Job drawing, mm, ordinate dimensions from the low corner. One solid piece. A direction names the side the tool comes from. Coordinates: 2 decimals unless noted, no trailing zeros. Loops run counter-clockwise (first coordinate to the right, second up) from the corner with the lowest first, then second, coordinate; pieces in that order, holes last. Notation, with made-up numbers: (-39.75, 4) -> (-19.75, 4) arc R12 cw to (-19.75, 24) -> close; hole circle Ø4 at (-22.5, -15). An arc over 180 degrees is marked (long way). Use one line per item in the form item = value. Start each with the question number.
(1) Band-saw the part on D-D on x = 99. Give the cut face in (y, z).
(2) Band-saw the part on C-C on y = 3.25. Give the cut face in (x, z).
(3) Pin check, flat tips, straight feed: P1, Ø6.5, axis at x = 32.5, y = 12.5, coming from the -Z side; P2, Ø5, axis at y = 7, z = 6, coming from the -X side; P3, Ø5, axis at y = 8, z = 2.5, coming from the +X side. Stop position of each tip, or through.
(4) Band-saw the part on B-B on x = 14. Give the cut face in (y, z).
(5) 3-axis set-ups, long thin cutter, end or side, ignore diameter. For the marked faces 1, 2 and 3: which of +Z, -Z, +X, -X, +Y, -Y reach the whole face in a straight line?
(6) Mould opens along X. For the marked faces 4, 5 and 6 say: +X half, -X half, draft (parallel to the pull), parting line (faces both ways), or undercut.
(7) Drill centre lines: L1, parallel to Z at x = 85.5, y = 18.5; L2, parallel to X at y = 15.5, z = 12.75; L3, parallel to Z at x = 104.5, y = 5.25. Where is each one in solid material? Low to high. Write a range as [from, to].
(8) Band-saw the part on A-A on z = 3.75. Give the cut face in (x, y).
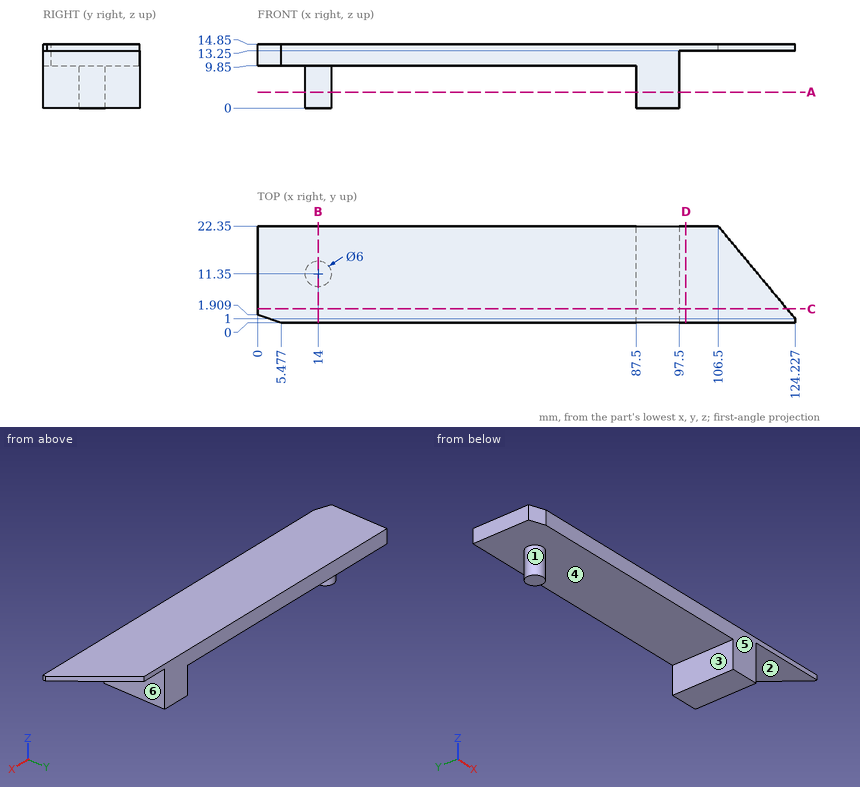
A:
q1.outline = (0, 13.25) -> (22.35, 13.25) -> (22.35, 14.85) -> (0, 14.85) -> close
q2.outline = (0, 9.85) -> (87.5, 9.85) -> (87.5, 0) -> (97.5, 0) -> (97.5, 13.25) -> (122.36, 13.25) -> (122.36, 14.85) -> (0, 14.85) -> close
q3.P1 = 9.85
q3.P2 = 11.64
q3.P3 = 97.5
q4.outline = (0, 9.85) -> (8.35, 9.85) -> (8.35, 0) -> (14.35, 0) -> (14.35, 9.85) -> (22.35, 9.85) -> (22.35, 14.85) -> (0, 14.85) -> close
q5.face_1 = -Z
q5.face_2 = -Z, +X, +Y, -Y
q5.face_3 = -Z, +Y, -Y
q6.face_4 = undercut
q6.face_5 = draft
q6.face_6 = +X half
q7.L1 = [9.85, 14.85]
q7.L2 = [0, 97.5]
q7.L3 = [13.25, 14.85]
q8.outline = circle Ø6 at (14, 11.35); (87.5, 0) -> (97.5, 0) -> (97.5, 22.35) -> (87.5, 22.35) -> close
